Part print with two shaded views. Sizes in mm from the minimum x, y, z corner. A direction names the side the tool comes from. Round coordinates to 2 decimals unless told otherwise and drop trailing zeros. Write each loop counter-clockwise with the first axis right and the second up, starting at its lowest first coordinate (ties: lowest second). Pieces come first, ordered by that corner, then holes. Notation, with made-up numbers: (63.5, 24) -> (114.5, 24) arc R30 ccw to (114.5, 61) -> close; hole circle Ø10 at (75, 1). An arc over 180 degrees is marked (long way). Return JSON: item names as keys, results as strings. Group by question number.
(1) Saw through at D-D (x = 3.2). List the corners of the cut face in (y, z) (3 decimals), plus the area to 4 significant figures.
(2) Drop a flat-ended pin along its axis: pin 1 Ø0.6 at (y, z) = (3.5, 3) entering from +X. Give the stop position or say it passes through.
(3) Drill centre lines: L1, parallel to Y at x = 5.7, z = 0.75; L2, parallel to Y at x = 3.2, z = 1.1 (3 decimals); L3, parallel to X at y = 1.8, z = 2.7 (3 decimals). Where is each one in solid material? Low to high. Write a range as from..to.
(4) Mould opens along X. For the marked faces 4, 5, 6 and 7 say: +X half, -X half, draft (parallel to the pull), parting line (faces both ways), or undercut.
(5) Saw through at B-B (x = 5.7). List the corners of the cut face in (y, z) (3 decimals).
(6) Tool access for the marked faces 1, 2 and 3: list every direction of +Z, -Z, +X, -X, +Y, -Y with a clear straight run to the whole face (end or side of a thin tool).
(7) Saw through at A-A (y = 1.5). List the corners of the cut face in (x, z) (3 decimals).
(8) Saw through at C-C (z = 4.4). List the corners of the cut face in (x, y) (3 decimals).
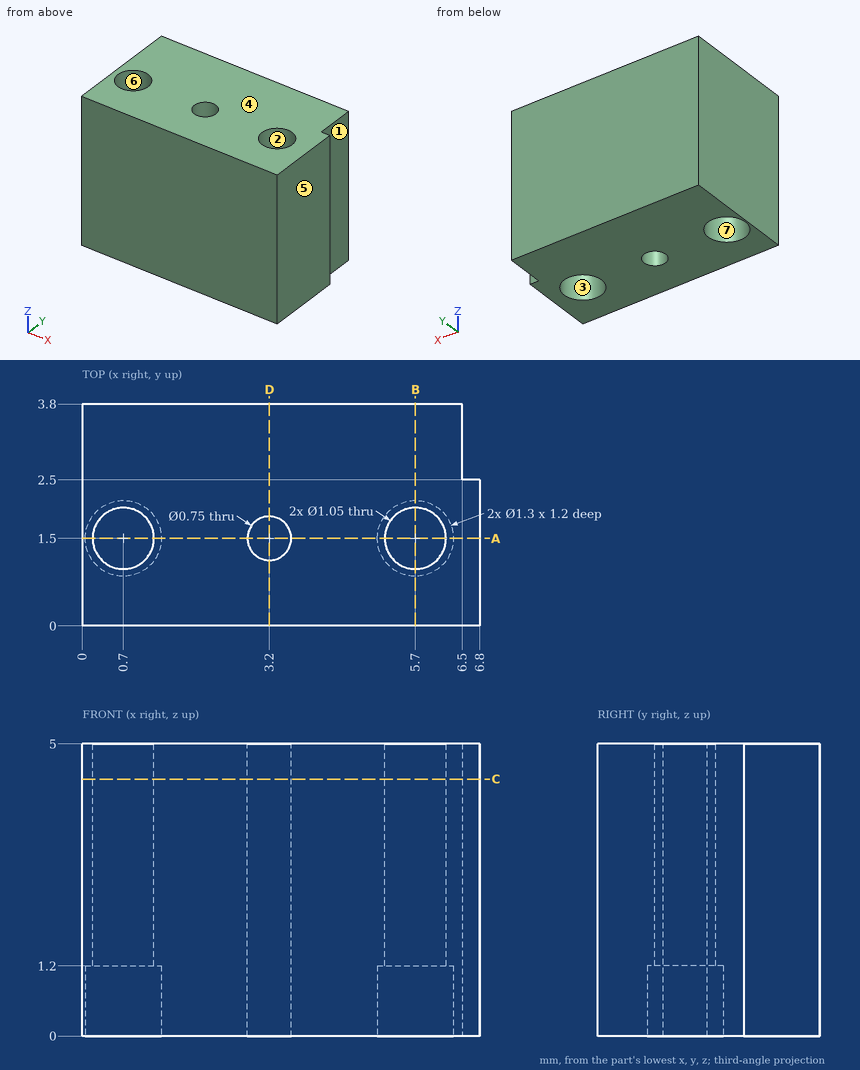
Computed values:
{
 "1": {"outline": "(0, 0) -> (1.125, 0) -> (1.125, 5) -> (0, 5) -> close; (1.875, 0) -> (3.8, 0) -> (3.8, 5) -> (1.875, 5) -> close", "area": "15.25 mm2"},
 "2": {"pin 1": "x = 6.5"},
 "3": {"L1": "0..0.85, 2.15..3.8", "L2": "0..1.125, 1.875..3.8", "L3": "0..0.269, 1.131..2.975, 3.425..5.269, 6.131..6.8"},
 "4": {"face 4": "draft", "face 5": "+X half", "face 6": "undercut", "face 7": "undercut"},
 "5": {"outline": "(0, 0) -> (0.85, 0) -> (0.85, 1.2) -> (0.975, 1.2) -> (0.975, 5) -> (0, 5) -> close; (2.025, 1.2) -> (2.15, 1.2) -> (2.15, 0) -> (3.8, 0) -> (3.8, 5) -> (2.025, 5) -> close"},
 "6": {"face 1": "+Z, -Z, +X, +Y", "face 2": "+Z, -Z", "face 3": "-Z"},
 "7": {"outline": "(0, 0) -> (0.05, 0) -> (0.05, 1.2) -> (0.175, 1.2) -> (0.175, 5) -> (0, 5) -> close; (1.225, 1.2) -> (1.35, 1.2) -> (1.35, 0) -> (2.825, 0) -> (2.825, 5) -> (1.225, 5) -> close; (3.575, 0) -> (5.05, 0) -> (5.05, 1.2) -> (5.175, 1.2) -> (5.175, 5) -> (3.575, 5) -> close; (6.225, 1.2) -> (6.35, 1.2) -> (6.35, 0) -> (6.8, 0) -> (6.8, 5) -> (6.225, 5) -> close"},
 "8": {"outline": "(0, 0) -> (6.8, 0) -> (6.8, 2.5) -> (6.5, 2.5) -> (6.5, 3.8) -> (0, 3.8) -> close; hole circle Ø1.05 at (0.7, 1.5); hole circle Ø0.75 at (3.2, 1.5); hole circle Ø1.05 at (5.7, 1.5)"}
}
